```python
from build123d import *

# Parameters (mm, degrees)
F0_R     = 2.5
F0_W     = 100
F0_H     = 5
F1_DEPTH = 5
F3_START = 36
F3_DEPTH = 14
F4_START = -36
F4_DEPTH = 14
F5_R     = 3.75
F6_DEPTH = 10
F8_DEPTH = 50


with BuildPart() as f1:
    # F0 (on Top) → F1 (new body)
    with BuildSketch(Plane.XY):
        with BuildLine():
            Line((50, 10), (-50, 10))
            Line((-50, 10), (-50, 0))
            Line((-50, 0), (-41.7705098312, 0))
            ThreePointArc((-41.7705098312, 0), (-25, 7.5), (-8.2294901688, 0))
            Line((-8.2294901688, 0), (8.2294901688, 0))
            ThreePointArc((8.2294901688, 0), (25, 7.5), (41.7705098312, 0))
            Line((41.7705098312, 0), (50, 0))
            Line((50, 0), (50, 10))
        make_face()
        with Locations((-45, 5)):
            Circle(F0_R, mode=Mode.SUBTRACT)
        with Locations((-5, 5)):
            Circle(F0_R, mode=Mode.SUBTRACT)
        with Locations((5, 5)):
            Circle(F0_R, mode=Mode.SUBTRACT)
        with Locations((45, 5)):
            Circle(F0_R, mode=Mode.SUBTRACT)
        with Locations((0, 12.5)):
            Rectangle(F0_W, F0_H)
    extrude(amount=F1_DEPTH)

    # F2 (on Right) → F3 (join)
    with BuildSketch(Plane.YZ.offset(F3_START)):
        Polygon((36.2132034356, -16.2132034356), (15, 5), (12.9289321881, 0), (32.6776695297, -19.7487373415), align=None)
        Polygon((43.2842712475, -23.2842712475), (36.2132034356, -16.2132034356), (32.6776695297, -19.7487373415), (22.0710678119, -30.3553390593), (29.1421356237, -37.4264068712), align=None)
    extrude(amount=F3_DEPTH)

    # F2 (on Right) → F4 (join)
    with BuildSketch(Plane.YZ.offset(F4_START)):
        Polygon((36.2132034356, -16.2132034356), (15, 5), (12.9289321881, 0), (32.6776695297, -19.7487373415), align=None)
        Polygon((43.2842712475, -23.2842712475), (36.2132034356, -16.2132034356), (32.6776695297, -19.7487373415), (22.0710678119, -30.3553390593), (29.1421356237, -37.4264068712), align=None)
    extrude(amount=-F4_DEPTH)

    # F5 (on face) → F6 (cut)
    with BuildSketch(Plane(origin=(0, 33.2842712475, -33.2842712475), x_dir=(-1, 0, 0), z_dir=(0, 0.7071067812, -0.7071067812))):
        with Locations((43, 1.1421356237)):
            Circle(F5_R)
        with Locations((-43, 1.1421356237)):
            Circle(F5_R)
    extrude(amount=-F6_DEPTH, mode=Mode.SUBTRACT)

    # F7 (on Right) → F8 (join, symmetric)
    with BuildSketch(Plane.YZ):
        Polygon((20, 0), (15, 5), (15, 0), align=None)
    extrude(amount=F8_DEPTH, both=True)


solid = f1.part
```
Here's how the part is built. I have some questions about the finished solid (model axes, mm). A direction names the side the tool comes from. Round coordinates to 2 decimals unless told otherwise and drop trailing zeros. Loops run counter-clockwise (first coordinate to the right, second up) from the corner with the lowest first, then second, coordinate; pieces in that order, holes last. Notation, with made-up numbers: (-1.5, 54) -> (30.5, 54) arc R22 cw to (30.5, 65) -> close; hole circle Ø7 at (40.25, 0). An arc over 180 degrees is marked (long way). Answer as CSV lines item,"result". Start each with the question number.
1. I need wall thicknesses on probe 1 along X at (y, z) = (36, -17); probe 2 along Y at (x, z) = (-45, 2); probe 3 along Y at (x, z) = (45, 3). Which ranges of each line are inside material? Lowest first, please. Write a range as from..to.
2. Imagine slicing it at A-A on x = 5. Write out the boundary of the cut face in (y, z).
3. If we mould it in two halves opening along Y, with no side actions, what happens to faces 4 (the face through (42.9, 22.67, -9.74)), 5 (the face through (-1, 9, 5)), 6 (the face through (47.31, 4.04, 2.46))? For each: pulls with the +Y half, pulls with the -Y half, needs draft (parallel to the pull), parting line crosses it, or undercut.
4. I'm going to push flat-ended pins straight in: P1, Ø16, axis at x = -12.5, y = 6, coming from the -Z side; P2, Ø4, axis at y = 29, z = -19.5, coming from the -X side; P3, Ø8, axis at x = 37.5, z = -25, coming from the -Y side. Where does each tip first touch, or does it pass through?
5. Imagine slicing it at D-D on x = -45. Write out the boundary of the cut face in (y, z), plus the area to 3 significant figures.
6. Imagine slicing it at C-C on y = 5. Write out the boundary of the cut face in (x, z).
7. Imagine slicing it at B-B on z = 2. Write out the boundary of the cut face in (x, y), plus the area to 3 significant figures.
8. For faces 1 (the face through (-1, 12, 0)), 2 (the face through (24.7, 7.5, 2.5)), 3 (the face through (-42.902, 29.806, -22.621)), which set-ups out of +Z, -Z, +X, -X, +Y, -Y let a thin tool reach every point of the face, with its end or its side?
Solution:
1,probe 1,"-50..-36, 36..50"
1,probe 2,"0..2.5, 7.5..18"
1,probe 3,"0..2.5, 7.5..17"
2,outline,"(0, 0) -> (2.5, 0) -> (2.5, 5) -> (0, 5) -> close; (7.5, 0) -> (20, 0) -> (15, 5) -> (7.5, 5) -> close"
3,face 4,"pulls with the -Y half"
3,face 5,"needs draft"
3,face 6,"undercut"
4,P1,"z = 0"
4,P2,"through"
4,P3,"y = 23.43"
5,outline,"(0, 0) -> (2.5, 0) -> (2.5, 5) -> (0, 5) -> close; (7.5, 0) -> (12.93, 0) -> (32.68, -19.75) -> (29.26, -23.16) -> (36.33, -30.23) -> (43.28, -23.28) -> (15, 5) -> (7.5, 5) -> close; (22.07, -30.36) -> (29.14, -37.43) -> (31.85, -34.72) -> (24.78, -27.65) -> close"
5,area,"326 mm²"
6,outline,"(-50, 0) -> (-47.5, 0) -> (-47.5, 5) -> (-50, 5) -> close; (-42.5, 0) -> (-35.31, 0) -> (-35.31, 5) -> (-42.5, 5) -> close; (-14.69, 0) -> (-7.5, 0) -> (-7.5, 5) -> (-14.69, 5) -> close; (-2.5, 0) -> (2.5, 0) -> (2.5, 5) -> (-2.5, 5) -> close; (7.5, 0) -> (14.69, 0) -> (14.69, 5) -> (7.5, 5) -> close; (35.31, 0) -> (42.5, 0) -> (42.5, 5) -> (35.31, 5) -> close; (47.5, 0) -> (50, 0) -> (50, 5) -> (47.5, 5) -> close"
7,outline,"(-50, 0) -> (-41.77, 0) arc R22.5 cw to (-8.23, 0) -> (8.23, 0) arc R22.5 cw to (41.77, 0) -> (50, 0) -> (50, 18) -> (-50, 18) -> close; hole circle Ø5 at (-45, 5); hole circle Ø5 at (-5, 5); hole circle Ø5 at (5, 5); hole circle Ø5 at (45, 5)"
7,area,"1,370 mm²"
8,face 1,"-Z, -Y"
8,face 2,"+Z, -Z, -Y"
8,face 3,"+X, -X, -Y"
